Can you work these out from the model? Positions are in its coordinate system, mm. A direction names the side the tool comes from. Round coordinates to 2 decimals unless told otherwise and drop trailing zeros. Loops run counter-clockwise (first coordinate to the right, second up) from the corner with the lowest first, then second, coordinate; pieces in that order, holes last. Notation, with made-up numbers: M 33,-20 L 74,-20 A19 ccw 74,-2 Z; hole C 30.25,67 d6. An arc over 180 degrees is marked long. Use a Markdown table: item, result. Add a question column.
```python
from build123d import *

# Parameters (mm, degrees)
SKETCH1_W               = 50.8
SKETCH1_H               = 50.8
BOSS_EXTRUDE1_DEPTH     = 13.97
F_1_4_CLEARANCE_HOLE1_D = 6.7564
SKETCH5_R               = 13.208
CUT_EXTRUDE1_DEPTH      = 1.5875
SKETCH6_R               = 3.81
CUT_EXTRUDE2_DEPTH      = 39.5419369
SKETCH10_R              = 6.858
CUT_EXTRUDE3_DEPTH      = 3.048
CUT_EXTRUDE4_START      = -6.858
SKETCH11_R              = 6.858
CUT_EXTRUDE4_DEPTH      = 6.858
SKETCH12_R              = 1.016
CUT_EXTRUDE5_DEPTH      = 19.05
CUT_EXTRUDE6_START      = -19.05
SKETCH13_R              = 1.016
CUT_EXTRUDE6_DEPTH      = 19.05


with BuildPart() as part:
    # Sketch1 → Boss-Extrude1 (new body)
    with BuildSketch(Plane(origin=(0, 0, 0), x_dir=(1, 0, 0), z_dir=(0, 1, 0))):
        Rectangle(SKETCH1_W, SKETCH1_H)
    extrude(amount=BOSS_EXTRUDE1_DEPTH)

    # 1/4 Clearance Hole1 (through all)
    with Locations(Plane(origin=(0, 13.97, 0), x_dir=(1, 0, 0), z_dir=(0, 1, 0))):
        with Locations((-20.6375, -20.6375), (-20.6375, 20.6375), (20.6375, 20.6375), (20.6375, -20.6375)):
            Hole(F_1_4_CLEARANCE_HOLE1_D / 2)

    # Sketch5 → Cut-Extrude1 (cut)
    with BuildSketch(Plane(origin=(0, 13.97, 0), x_dir=(1, 0, 0), z_dir=(0, 1, 0))):
        with Locations(Location((0, 0, 0), (0, 0, 270))):
            Circle(SKETCH5_R)
    extrude(amount=-CUT_EXTRUDE1_DEPTH, mode=Mode.SUBTRACT)

    # Sketch6 → Cut-Extrude2 (cut, through all)
    with BuildSketch(Plane(origin=(0, 13.97, 0), x_dir=(1, 0, 0), z_dir=(0, 1, 0))):
        with Locations(Location((0, 20.32, 0), (0, 0, 270))):
            Circle(SKETCH6_R)
        with Locations(Location((20.32, 0, 0), (0, 0, 270))):
            Circle(SKETCH6_R)
        with Locations(Location((0, -20.32, 0), (0, 0, 270))):
            Circle(SKETCH6_R)
        with Locations(Location((-20.32, 0, 0), (0, 0, 270))):
            Circle(SKETCH6_R)
    extrude(amount=-CUT_EXTRUDE2_DEPTH, mode=Mode.SUBTRACT)

    # Sketch10 → Cut-Extrude3 (cut)
    with BuildSketch(Plane(origin=(0, 13.97, 0), x_dir=(1, 0, 0), z_dir=(0, 1, 0))):
        with Locations((-20.32, 0)):
            Circle(SKETCH10_R)
        with Locations((0, 20.32)):
            Circle(SKETCH10_R)
        with Locations((20.32, 0)):
            Circle(SKETCH10_R)
        with Locations((0, -20.32)):
            Circle(SKETCH10_R)
    extrude(amount=-CUT_EXTRUDE3_DEPTH, mode=Mode.SUBTRACT)

    # Sketch11 → Cut-Extrude4 (cut)
    with BuildSketch(Plane.XZ.offset(CUT_EXTRUDE4_START)):
        with Locations((-20.32, 0)):
            Circle(SKETCH11_R)
        with Locations((0, 20.32)):
            Circle(SKETCH11_R)
        with Locations((20.32, 0)):
            Circle(SKETCH11_R)
        with Locations((0, -20.32)):
            Circle(SKETCH11_R)
    extrude(amount=CUT_EXTRUDE4_DEPTH, mode=Mode.SUBTRACT)

    # Sketch12 → Cut-Extrude5 (cut)
    with BuildSketch(Plane.XY.offset(25.4)):
        with Locations((8.417142715, 10.795)):
            Circle(SKETCH12_R)
    extrude(amount=-CUT_EXTRUDE5_DEPTH, mode=Mode.SUBTRACT)

    # Sketch13 → Cut-Extrude6 (cut)
    with BuildSketch(Plane(origin=(0, 0, -25.4), x_dir=(-1, 0, 0), z_dir=(0, 0, -1)).offset(CUT_EXTRUDE6_START)):
        with Locations(Location((-8.417142715, 10.795, 0), (0, 0, 180))):
            Circle(SKETCH13_R)
    extrude(amount=CUT_EXTRUDE6_DEPTH, mode=Mode.SUBTRACT)


solid = part.part
```
(1) On a 3-axis mill with a long thin cutter (end or side, diameter ignored), from which of +Z, -Z, +X, -X, +Y, -Y can I reach the whole of each face in a straight line? I mean faces 1 (the face through (8, 11, 6.35)), 2 (the face through (-0.231, 3.477, 13.466)), 3 (the face through (0, 12.382, 0)). Say none if no direction works.
(2) If I drill on probe 1 along X at (y, z) = (5, 20.5); probe 2 along X at (y, z) = (9.65, 20.32); probe 3 along Z at (x, y) = (21, 10.5), over which ranges is the centre line in solid material (lowest first)? Write a range as [from, to].
(3) Suppose I cut it at B-B on z = 0. List the corners of the cut face in (x, y) for me, and give its area (3 significant figures).
(4) Suppose I cut it at D-D on x = -18. List the corners of the cut face in (y, z) for me.
(5) Thinking about a two-plate mould opening in Y: for faces 4 (the face through (16.69, 10.922, -1.62)), 5 (the face through (0, 8, -25.4)), 6 (the face through (9.386, 11.1, 16.008)), which applies, released by +Y, released by -Y, zero draft, split by the parting line, or undercut?
(6) I'm going to push flat-ended pins straight in: pin 1 (11 mm diameter, centred on x = -20.64, z = 20.64, fed in from +Y); pin 2 (11 mm diameter, centred on x = 0, z = 20.32, fed in from -Y); pin 3 (4.5 mm diameter, centred on x = -20.32, z = 0, fed in from -Y); pin 4 (3.5 mm diameter, centred on x = -22.5, z = -1.5, fed in from +Y). Where does each tip first touch, or does it pass through?
(7) Suppose I cut it at C-C on z = -19.5. List the corners of the cut face in (x, y) for me (3 decimals).
(8) Suppose I cut it at A-A on x = 0. List the corners of the cut face in (y, z) for me.
Results below:
| question | item | result |
|---|---|---|
| 1 | face 1 | +Z |
| 1 | face 2 | -Y |
| 1 | face 3 | +Y |
| 2 | probe 1 | x = [-25.4, -24.01], [-17.26, -6.86], [6.86, 17.26], [24.01, 25.4] |
| 2 | probe 2 | x = [-25.4, -24], [-17.27, -3.81], [3.81, 17.27], [24, 25.4] |
| 2 | probe 3 | z = [-25.4, -24], [-17.28, -3.75], [3.75, 17.28], [24, 25.4] |
| 3 | outline | M -25.4,6.86 L -24.13,6.86 L -24.13,10.92 L -25.4,10.92 Z; M -16.51,6.86 L -13.46,6.86 L -13.46,0 L 13.46,0 L 13.46,6.86 L 16.51,6.86 L 16.51,10.92 L 13.46,10.92 L 13.46,13.97 L 13.21,13.97 L 13.21,12.38 L -13.21,12.38 L -13.21,13.97 L -13.46,13.97 L -13.46,10.92 L -16.51,10.92 Z; M 24.13,6.86 L 25.4,6.86 L 25.4,10.92 L 24.13,10.92 Z |
| 3 | area | 369 mm² |
| 4 | outline | M 0,-25.4 L 13.97,-25.4 L 13.97,-22.75 L 0,-22.75 Z; M 0,-18.53 L 13.97,-18.53 L 13.97,-6.45 L 10.92,-6.45 L 10.92,-3.02 L 6.86,-3.02 L 6.86,-6.45 L 0,-6.45 Z; M 0,6.45 L 6.86,6.45 L 6.86,3.02 L 10.92,3.02 L 10.92,6.45 L 13.97,6.45 L 13.97,18.53 L 0,18.53 Z; M 0,22.75 L 13.97,22.75 L 13.97,25.4 L 0,25.4 Z |
| 5 | face 4 | released by +Y |
| 5 | face 5 | zero draft |
| 5 | face 6 | undercut |
| 6 | pin 1 | stops at y = 13.97 |
| 6 | pin 2 | stops at y = 6.86 |
| 6 | pin 3 | passes through |
| 6 | pin 4 | stops at y = 10.92 |
| 7 | outline | M -25.4,0 L -23.818,0 L -23.818,13.97 L -25.4,13.97 Z; M -17.457,0 L -6.809,0 L -6.809,6.858 L -3.721,6.858 L -3.721,10.922 L -6.809,10.922 L -6.809,13.97 L -17.457,13.97 Z; M 3.721,6.858 L 6.809,6.858 L 6.809,0 L 17.457,0 L 17.457,13.97 L 6.809,13.97 L 6.809,10.922 L 3.721,10.922 Z; M 23.818,0 L 25.4,0 L 25.4,13.97 L 23.818,13.97 Z; hole C 8.417,10.795 d2.032 |
| 8 | outline | M 0,-13.46 L 6.86,-13.46 L 6.86,-16.51 L 10.92,-16.51 L 10.92,-13.46 L 13.97,-13.46 L 13.97,-13.21 L 12.38,-13.21 L 12.38,13.21 L 13.97,13.21 L 13.97,13.46 L 10.92,13.46 L 10.92,16.51 L 6.86,16.51 L 6.86,13.46 L 0,13.46 Z; M 6.86,-25.4 L 10.92,-25.4 L 10.92,-24.13 L 6.86,-24.13 Z; M 6.86,24.13 L 10.92,24.13 L 10.92,25.4 L 6.86,25.4 Z |
